Design review of the part built by this model. Coordinates are the model's own, in mm. A direction names the side the tool comes from. Give positions to 0.01 mm unless a question says otherwise; leave off trailing zeros. Write each loop counter-clockwise with the first axis right and the second up, starting at its lowest first coordinate (ties: lowest second). Pieces come first, ordered by that corner, then holes. Notation, with made-up numbers: M -34,47.25 L 15,47.25 A22 ccw 15,65.25 Z; hole C 49.25,31 d2. An arc over 180 degrees is marked long. One line per item, written item: value. Start each with the question number.
```python
from build123d import *

# Parameters (mm, degrees)
SKETCH1_R                       = 1
BOSS_EXTRUDE1_DEPTH             = 6
FILLET1_R                       = 4
FILLET2_R                       = 4
M3X0_5_TAPPED_HOLE1_D           = 2.5
M3X0_5_TAPPED_HOLE1_DEPTH       = 4
M3X0_5_TAPPED_HOLE1_CSINK_D     = 3.05
M3X0_5_TAPPED_HOLE1_CSINK_ANGLE = 90
M3X0_5_TAPPED_HOLE1_TIP         = 0.751075774
F_2_0_2_DIAMETER_HOLE1_D        = 2
F_2_0_2_DIAMETER_HOLE1_DEPTH    = 3
F_2_0_2_DIAMETER_HOLE1_TIP      = 0.600860619
SKETCH8_R                       = 3
CUT_EXTRUDE1_DEPTH              = 3
SKETCH9_R                       = 1.5
CUT_EXTRUDE2_DEPTH              = 4


with BuildPart() as part:
    # Sketch1 → Boss-Extrude1 (new body)
    with BuildSketch(Plane.XY):
        Polygon((-27.266838493, 36), (-30.5, 30.4), (-30.5, 26), (-30.5, 20), (-16, 20), (-16, 8), (-16, 0), (0, 0), (0, 8), (-8, 8), (-8, 26), (-16, 26), (-23.5, 26), (-23.5, 36), align=None)
        with Locations((-28.55, 28.91)):
            Circle(SKETCH1_R, mode=Mode.SUBTRACT)
        with Locations((-25.55, 34.106152423)):
            Circle(SKETCH1_R, mode=Mode.SUBTRACT)
    extrude(amount=BOSS_EXTRUDE1_DEPTH)

    # Fillet1
    fillet1_edges = [part.edges().sort_by_distance(p)[0] for p in [
        (-23.5, 26, 3),
    ]]
    fillet(fillet1_edges, radius=FILLET1_R)

    # Fillet2
    fillet2_edges = [part.edges().sort_by_distance(p)[0] for p in [
        (-8, 8, 3),
    ]]
    fillet(fillet2_edges, radius=FILLET2_R)

    # M3x0.5 Tapped Hole1
    with Locations(Plane(origin=(0, 0, 0), x_dir=(-1, 0, 0), z_dir=(0, -1, 0))):
        with Locations((13, -3), (3, -3)):
            CounterSinkHole(M3X0_5_TAPPED_HOLE1_D / 2, M3X0_5_TAPPED_HOLE1_CSINK_D / 2, depth=M3X0_5_TAPPED_HOLE1_DEPTH, counter_sink_angle=M3X0_5_TAPPED_HOLE1_CSINK_ANGLE)
            with Locations((0, 0, -(M3X0_5_TAPPED_HOLE1_DEPTH + M3X0_5_TAPPED_HOLE1_TIP / 2))):  # 118° drill point
                Cone(0, M3X0_5_TAPPED_HOLE1_D / 2, M3X0_5_TAPPED_HOLE1_TIP, mode=Mode.SUBTRACT)

    # Ø2.0 (2) Diameter Hole1
    with Locations(Plane(origin=(0, 0, 0), x_dir=(-1, 0, 0), z_dir=(0, -1, 0))):
        with Locations((8, -3)):
            Hole(F_2_0_2_DIAMETER_HOLE1_D / 2, depth=F_2_0_2_DIAMETER_HOLE1_DEPTH)
            with Locations((0, 0, -(F_2_0_2_DIAMETER_HOLE1_DEPTH + F_2_0_2_DIAMETER_HOLE1_TIP / 2))):  # 118° drill point
                Cone(0, F_2_0_2_DIAMETER_HOLE1_D / 2, F_2_0_2_DIAMETER_HOLE1_TIP, mode=Mode.SUBTRACT)

    # Sketch8 → Cut-Extrude1 (cut)
    with BuildSketch(Plane(origin=(0, 0, 0), x_dir=(-1, 0, 0), z_dir=(0, 0, -1))):
        with Locations((12, 22)):
            Circle(SKETCH8_R)
        with Locations((12, 8)):
            Circle(SKETCH8_R)
    extrude(amount=-CUT_EXTRUDE1_DEPTH, mode=Mode.SUBTRACT)

    # Sketch9 → Cut-Extrude2 (cut, through all)
    with BuildSketch(Plane(origin=(0, 0, 3), x_dir=(-1, 0, 0), z_dir=(0, 0, -1))):
        with Locations((12, 22)):
            Circle(SKETCH9_R)
        with Locations((12, 8)):
            Circle(SKETCH9_R)
    extrude(amount=-CUT_EXTRUDE2_DEPTH, mode=Mode.SUBTRACT)


solid = part.part
```
Q1. For P1, Ø5, axis at x = -12, y = 22, coming from the +Z side; P2, Ø3, axis at x = -13, z = 3, coming from the +Y side; P3, Ø3, axis at x = -20, z = 3.5, coming from the -Y side; P4, Ø5.5, axis at x = -12, y = 8, coming from the -Z side, all flat-tipped, find the tip position at first contact; note any pin that passes through.
Q2. Take a section at D-D, the plane y = 6. Give the boundary of the cut face in (x, z), then the cut area to 3 significant figures.
Q3. Wall thickness on line 1 (Y direction, x = -12, z = 1.7); line 2 (Y direction, x = -12, z = 4.2); line 3 (Z direction, x = -3, y = 2): over which ranges is each line inside the solid? List them lowest first. Write a range as from..to.
Q4. Machinability: for faces 4 (the face through (-8.8, 1.5, 3.6)), 5 (the face through (-23, 20, 3)), 6 (the face through (-13.3, 6.7, 3)), which of the approach directions +Z, -Z, +X, -X, +Y, -Y give a long, thin tool a straight path to every point of the face, cutting with its end or side? Answer none if there is none.
Q5. Take a section at C-C, the plane z = 5.3. Give the boundary of the cut face in (x, y).
Q6. The part is to be moulded in two halves that separate along X. For faces 1 (the face through (-13.3, 20.7, 3)), 2 (the face through (-22.359, 27.203, 3.042)), 3 (the face through (-30.5, 25, 3)), say which applies: pulls with the +X half, pulls with the -X half, needs draft (parallel to the pull), parting line crosses it, or undercut.
Q7. Take a section at A-A, the plane x = -25.55. Give the boundary of the cut face in (y, z), then the cut area to 3 significant figures.
Q8. Take a section at B-B, the plane y = 33.5. Give the boundary of the cut face in (x, z), then the cut area to 3 significant figures.
Results list:
1. P1: stops at z = 6
1. P2: stops at y = 26
1. P3: stops at y = 20
1. P4: stops at z = 3
2. outline: M -16,0 L -14.24,0 L -14.24,3 L -9.76,3 L -9.76,0 L 0,0 L 0,6 L -16,6 Z
2. area: 82.6 mm^2
3. line 1: y = 0..5, 11..19, 25..26
3. line 2: y = 0..6.5, 9.5..20.5, 23.5..26
3. line 3: z = 0..1.75, 4.25..6
4. face 4: -Y
4. face 5: +Z, -Z, -X, -Y
4. face 6: -Z
5. outline: M -30.5,20 L -16,20 L -16,0 L 0,0 L 0,8 L -4,8 A4 cw -8,12 L -8,26 L -19.5,26 A4 cw -23.5,30 L -23.5,36 L -27.27,36 L -30.5,30.4 Z; hole C -28.55,28.91 d2; hole C -25.55,34.11 d2; hole C -12,8 d3; hole C -12,22 d3
6. face 1: undercut
6. face 2: pulls with the +X half
6. face 3: pulls with the -X half
7. outline: M 20,0 L 33.11,0 L 33.11,6 L 20,6 Z; M 35.11,0 L 36,0 L 36,6 L 35.11,6 Z
7. area: 84.0 mm^2
8. outline: M -28.71,0 L -26.35,0 L -26.35,6 L -28.71,6 Z; M -24.75,0 L -23.5,0 L -23.5,6 L -24.75,6 Z
8. area: 21.7 mm^2
